Autodesk Inventor part; units mm, degrees
ref_plane "YZ Plane" through (0, 0, 0) normal (1, 0, 0) x (0, 1, 0)
ref_plane "XZ Plane" through (0, 0, 0) normal (0, 1, 0) x (-1, 0, 0)
ref_plane "XY Plane" through (0, 0, 0) normal (0, 0, 1) x (1, 0, 0)
sketch "Sketch1" plane through (0, 0, 0) normal (0, 1, 0) x (-1, 0, 0)
  circle A0 centre (-31.75, 0) radius 11.0744
  circle A1 centre (24.765, 0) radius 9.652
  line L0 (-4.3934, -6.35) -> (0.9525, -6.35)
  arc A2 (16.1925, -11.43) -> (16.1925, 11.43) centre (24.765, 0) ccw
  arc A3 (-20.9731, 12.5076) -> (-20.9731, -12.5076) centre (-31.75, 0) ccw
  line L1 (-4.3934, 6.35) -> (0.9525, 6.35)
  line L2 (-54.5659, 23.0342) -> (48.7426, 23.0342)
  line L3 (48.7426, 23.0342) -> (48.7426, -24.079)
  line L4 (48.7426, -24.079) -> (-54.5659, -24.079)
  line L5 (-54.5659, -24.079) -> (-54.5659, 23.0342)
  arc A4 (-20.9731, 12.5076) -> (-4.3934, 6.35) centre (-4.3934, 31.75) ccw
  arc A5 (0.9525, 6.35) -> (16.1925, 11.43) centre (0.9525, 31.75) ccw
  arc A6 (16.1925, -11.43) -> (0.9525, -6.35) centre (0.9525, -31.75) ccw
  arc A7 (-4.3934, -6.35) -> (-20.9731, -12.5076) centre (-4.3934, -31.75) ccw
  arc A8 (0.9525, 6.729) -> (15.9651, 11.7332) centre (0.9525, 31.75) ccw
  line L6 (0.9525, 6.729) -> (-4.3934, 6.729)
  arc A9 (-20.7258, 12.7947) -> (-4.3934, 6.729) centre (-4.3934, 31.75) ccw
  arc A10 (-20.7258, 12.7947) -> (-20.7258, -12.7947) centre (-31.75, 0) ccw
  arc A11 (-4.3934, -6.729) -> (-20.7258, -12.7947) centre (-4.3934, -31.75) ccw
  line L7 (-4.3934, -6.729) -> (0.9525, -6.729)
  arc A12 (15.9651, -11.7332) -> (0.9525, -6.729) centre (0.9525, -31.75) ccw
  arc A13 (15.9651, -11.7332) -> (15.9651, 11.7332) centre (24.765, 0) ccw
  circle A14 centre (24.765, 0) radius 0.7937
  circle A15 centre (-31.75, 0) radius 0.7938
  point P0 (0, 0)
  point P1 (-16.51, -6.35)
  point P2 (-16.51, 6.35)
  point P3 (11.9662, -6.35)
  point P4 (11.9662, 6.35)
  dimension "d15" = 22.1488
  dimension "d17" = 12.7
  dimension "d18" = 33.02
  dimension "d19" = 19.304
  dimension "d20" = 28.575
  dimension "d21" = 56.515
  dimension "d35" = 25.4
  dimension "d40" = 1.5875
  dimension "d41" = 1.5875
extrude "Extrusion3" add sketch "Sketch1" against normal blind 25.4 contours A0 | A1 | A7 A3 A4 L1 A5 A2 A6 L0 | L2 L3 L4 L5 | A8 A13 A12 L7 A11 A10 A9 L6 | A14 | A15
extrude "Extrusion4" cut sketch "Sketch1" against normal blind 7.874 contours A0 | A1 | A7 A3 A4 L1 A5 A2 A6 L0 | A8 A13 A12 L7 A11 A10 A9 L6 | A14 | A15
extrude "Extrusion5" cut sketch "Sketch1" against normal blind 254 contours A14 | A15
properties part number "C.Connecting Rod Cutting Jig"
Here's how the part is built. I have some questions about the finished solid (model axes, mm). A direction names the side the tool comes from. Coordinates: 2 decimals unless noted, no trailing zeros. Write each loop counter-clockwise with the first axis right and the second up, starting at its lowest first coordinate (ties: lowest second). Pieces come first, ordered by that corner, then holes. Notation, with made-up numbers: (36.25, 40) - (85.25, 40) arc R24 ccw to (85.25, 60) - close; hole circle Ø9 at (-7.75, 6). An arc over 180 degrees is marked (long way). Use one line per item in the form item = value.
1) On a 3-axis mill with a long thin cutter (end or side, diameter ignored), from which of +Z, -Z, +X, -X, +Y, -Y can I reach the whole of each face in a straight line? I mean faces 4 (the cylindrical face through (12.988, -3.882, -8.251)), 5 (the flat face through (4, -25.4, 0)). Say none if no direction works.
Solved:
face_4 = +Y
face_5 = +Z, -Z, +X, -X, -Y
2) Suppose I cut it at A-A, the plane z = 2. Write out the boundary of the cut face in (x, y), plus the area to 3 significant figures.
Solved:
outline = (-48.74, -25.4) - (54.57, -25.4) - (54.57, 0) - (48.52, 0) - (48.52, -7.87) - (-39.29, -7.87) - (-39.29, 0) - (-48.74, 0) - close
area = 1,930 mm2
3) I'm going to push a flat-ended pin straight in: P1, Ø12, axis at x = -22, z = 5.5, coming from the +Y side. Where does the tip first touch, or does it pass through?
Solved:
P1 = -7.87
4) Suppose I cut it at C-C, the plane z = -9.5. Write out the boundary of the cut face in (x, y), plus the area to 3 significant figures.
Solved:
outline = (-48.74, -25.4) - (54.57, -25.4) - (54.57, 0) - (45.71, 0) - (45.71, -7.87) - (15.84, -7.87) - (15.84, 0) - (-12.4, 0) - (-12.4, -7.87) - (-35.94, -7.87) - (-35.94, 0) - (-48.74, 0) - close
area = 2,200 mm2
5) I need wall thicknesses on line 1 (X direction, y = -2.5, z = 0); line 2 (Z direction, x = 31.75, y = -3.25); line 3 (Z direction, x = 31.75, y = -21.5). Which ranges of each line are inside material? Lowest first, please.
Solved:
line_1 = -48.74 to -39.43, 48.64 to 54.57
line_2 = -24.08 to -16.89, 16.89 to 23.03
line_3 = -24.08 to -0.79, 0.79 to 23.03
6) Suppose I cut it at B-B, the plane x = 40.5. Write out the boundary of the cut face in (y, z).
Solved:
outline = (-25.4, -24.08) - (0, -24.08) - (0, -14.45) - (-7.87, -14.45) - (-7.87, 14.45) - (0, 14.45) - (0, 23.03) - (-25.4, 23.03) - close
7) Thinking about a two-plate mould opening in Z: for faces 1 (the flat face through (2, -13, -24.079)), 2 (the cylindrical face through (48.63, -3.88, 0.54)), 3 (the flat face through (54.566, -13, -1)), which applies, released by +Z, released by -Z, zero draft, split by the parting line, or undercut?
Solved:
face_1 = released by -Z
face_2 = undercut
face_3 = zero draft
